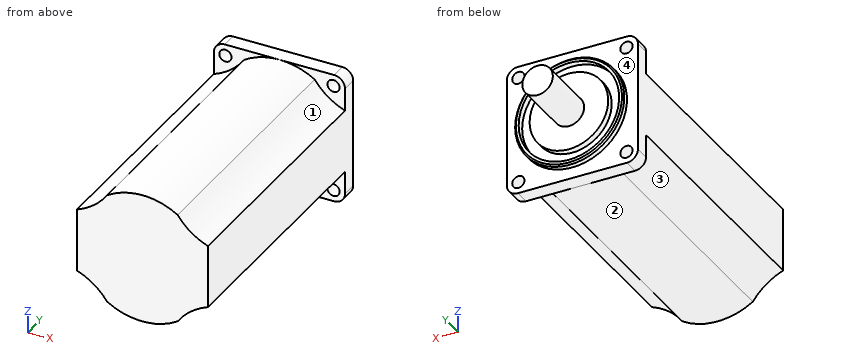
from build123d import *

# Parameters (mm, degrees)
SKETCH1_R           = 2.8
BOSS_EXTRUDE1_DEPTH = 7
SKETCH2_R           = 25
SKETCH2_R_2         = 23
SKETCH2_R_3         = 18
BOSS_EXTRUDE3_DEPTH = 3
CHAMFER2_SIZE       = 0.71
BOSS_EXTRUDE4_DEPTH = 118
SKETCH5_R           = 7
BOSS_EXTRUDE5_DEPTH = 27


with BuildPart() as part:
    # Sketch1 → Boss-Extrude1 (new body)
    with BuildSketch(Plane(origin=(0, 0, 0), x_dir=(1, 0, 0), z_dir=(0, 1, 0))):
        with BuildLine():
            Line((-25, -30), (25, -30))
            ThreePointArc((25, -30), (28.535533906, -28.535533906), (30, -25))
            Line((30, -25), (30, 25))
            ThreePointArc((30, 25), (28.535533906, 28.535533906), (25, 30))
            Line((25, 30), (-25, 30))
            ThreePointArc((-25, 30), (-28.535533906, 28.535533906), (-30, 25))
            Line((-30, 25), (-30, -25))
            ThreePointArc((-30, -25), (-28.535533906, -28.535533906), (-25, -30))
        make_face()
        with Locations((-24.748737342, 24.748737342)):
            Circle(SKETCH1_R, mode=Mode.SUBTRACT)
        with Locations((24.748737342, 24.748737342)):
            Circle(SKETCH1_R, mode=Mode.SUBTRACT)
        with Locations((24.748737342, -24.748737342)):
            Circle(SKETCH1_R, mode=Mode.SUBTRACT)
        with Locations((-24.748737342, -24.748737342)):
            Circle(SKETCH1_R, mode=Mode.SUBTRACT)
    extrude(amount=BOSS_EXTRUDE1_DEPTH)

    # Sketch2 → Boss-Extrude3 (add)
    with BuildSketch(Plane(origin=(0, 7, 0), x_dir=(1, 0, 0), z_dir=(0, 1, 0))):
        Circle(SKETCH2_R)
        Circle(SKETCH2_R_2, mode=Mode.SUBTRACT)
        Circle(SKETCH2_R_3)
    extrude(amount=BOSS_EXTRUDE3_DEPTH)

    # Chamfer2
    chamfer2_edges = [part.edges().sort_by_distance(p)[0] for p in [
        (-25, 10, 0),
    ]]
    chamfer(chamfer2_edges, length=CHAMFER2_SIZE)

    # Sketch3 → Boss-Extrude4 (add)
    with BuildSketch(Plane.XZ):
        with BuildLine():
            Line((-30, 14.5), (-30, -14.5))
            ThreePointArc((-30, -14.5), (-22.221450139, -18.82296717), (-16.12, -25.30109879))
            ThreePointArc((-16.12, -25.30109879), (0, -30), (16.12, -25.30109879))
            ThreePointArc((16.12, -25.30109879), (22.221450139, -18.82296717), (30, -14.5))
            Line((30, -14.5), (30, 14.5))
            ThreePointArc((30, 14.5), (22.221450139, 18.82296717), (16.12, 25.30109879))
            ThreePointArc((16.12, 25.30109879), (0, 30), (-16.12, 25.30109879))
            ThreePointArc((-16.12, 25.30109879), (-22.221450139, 18.82296717), (-30, 14.5))
        make_face()
    extrude(amount=BOSS_EXTRUDE4_DEPTH)

    # Sketch5 → Boss-Extrude5 (add)
    with BuildSketch(Plane(origin=(0, 10, 0), x_dir=(1, 0, 0), z_dir=(0, 1, 0))):
        Circle(SKETCH5_R)
    extrude(amount=BOSS_EXTRUDE5_DEPTH)


solid = part.part
Design review of the part built by this model. Coordinates are the model's own, in mm. Face numbers are marked on the shaded views. A direction names the side the tool comes from. Coordinates: 2 decimals unless noted, no trailing zeros. Loops run counter-clockwise (first coordinate to the right, second up) from the corner with the lowest first, then second, coordinate; pieces in that order, holes last. Notation, with made-up numbers: M -5.75,88.25 L 13.25,88.25 A33 cw 13.25,117.25 Z; hole C 7.25,44 d3. An arc over 180 degrees is marked long. Use one line per item in the form item = value.
(1) Consider section A-A (y = -92.5). Write out the cut boundary in (x, z).
Return value:
outline = M -30,-14.5 A29 cw -16.12,-25.3 A30 ccw 16.12,-25.3 A29 cw 30,-14.5 L 30,14.5 A29 cw 16.12,25.3 A30 ccw -16.12,25.3 A29 cw -30,14.5 Z
(2) Consider section B-B (z = 0). Write out the cut boundary in (x, y).
Return value:
outline = M -30,-118 L 30,-118 L 30,7 L 25,7 L 25,9.29 L 24.29,10 L 23,10 L 23,7 L 18,7 L 18,10 L 7,10 L 7,37 L -7,37 L -7,10 L -18,10 L -18,7 L -23,7 L -23,10 L -24.29,10 L -25,9.29 L -25,7 L -30,7 Z
(3) Clearance check with flat-ended pins moving along their axes: P1, Ø10, axis at x = -12.5, y = -35, coming from the +Z side; P2, Ø1, axis at x = 11, y = -18, coming from the +Z side; P3, Ø5, axis at x = -1, y = -7.5, coming from the -Z side; P4, Ø8, axis at x = -15, y = -8, coming from the +Z side. State where each tip first meets the part, or that it passes through.
Return value:
P1 = 29.05
P2 = 28.1
P3 = -30
P4 = 27.91
(4) For the marked faces 1, 2, 3 and 4, list the 3-axis set-ups (+Z, -Z, +X, -X, +Y, -Y) from which the entire face can be reached by the end or side of a thin tool; tool diameter is ignored.
Return value:
face_1 = +Z, +X, -Y
face_2 = -Z, -Y
face_3 = -Z, -X, -Y
face_4 = +Y
(5) Consider section C-C (y = 4). Write out the cut boundary in (x, z).
Return value:
outline = M -30,-25 A5 ccw -25,-30 L 25,-30 A5 ccw 30,-25 L 30,25 A5 ccw 25,30 L -25,30 A5 ccw -30,25 Z; hole C -24.75,-24.75 d5.6; hole C -24.75,24.75 d5.6; hole C 24.75,-24.75 d5.6; hole C 24.75,24.75 d5.6
(6) For line 1 along X through (y, z) = (9.3, 0); line 2 along Z through (x, y) = (0, 9.15); line 3 along Y through (x, z) = (27.5, 27), list the stretches that pass through material, from the lowest coordinate up. Write a range as from..to.
Return value:
line_1 = -24.99..-23, -18..18, 23..24.99
line_2 = -25..-23, -18..18, 23..25
line_3 = 0..7
